Check sheet for the modelled part. Datum: model origin and axes. Units: mm. Face numbers are marked on the shaded views. A direction names the side the tool comes from. Give positions to 0.01 mm unless a question says otherwise; leave off trailing zeros. Order: outer loops, then holes, each group sorted by start corner. A loop starts at its lowest first (then second) coordinate and runs counter-clockwise, first axis right, second up.
from build123d import *

# Parameters (mm, degrees)
F0_R      = 2.25
F0_R_2    = 1
F1_DEPTH  = 4
F2_W      = 12
F2_H      = 12
F2_R      = 2.25
F3_DEPTH  = 6
F4_W      = 8
F4_H      = 8
F5_DEPTH  = 2
F6_R      = 4
F6_R_2    = 2.25
F7_DEPTH  = 5
F8_R      = 2.5
F8_R_2    = 1
F9_DEPTH  = 4
F11_DEPTH = 4.001


with BuildPart() as f1:
    # F0 (on Top) → F1 (new body)
    with BuildSketch(Plane.XY):
        Polygon((-30, 46), (-42, 46), (-42, -46), (-30, -46), (-30, -34), (13, -34), (13, -46), (25, -46), (25, -34), (40, -34), (40, 34), (25, 34), (25, 46), (13, 46), (13, 34), (-30, 34), align=None)
        with Locations((-36, -40)):
            Circle(F0_R, mode=Mode.SUBTRACT)
        with Locations((-30, -28)):
            Circle(F0_R_2, mode=Mode.SUBTRACT)
        with Locations((19, -40)):
            Circle(F0_R, mode=Mode.SUBTRACT)
        with Locations((28, -28)):
            Circle(F0_R_2, mode=Mode.SUBTRACT)
        with Locations((-30, 21)):
            Circle(F0_R_2, mode=Mode.SUBTRACT)
        with Locations((-36, 40)):
            Circle(F0_R, mode=Mode.SUBTRACT)
        with Locations((28, 21)):
            Circle(F0_R_2, mode=Mode.SUBTRACT)
        with Locations((19, 40)):
            Circle(F0_R, mode=Mode.SUBTRACT)
    extrude(amount=F1_DEPTH)

    # F2 (on face) → F3 (join)
    with BuildSketch(Plane.XY.offset(4)):
        with Locations((-36, -40)):
            Rectangle(F2_W, F2_H)
        with Locations((-36, -40)):
            Circle(F2_R, mode=Mode.SUBTRACT)
        with Locations((-36, 40)):
            Rectangle(F2_W, F2_H)
        with Locations((-36, 40)):
            Circle(F2_R, mode=Mode.SUBTRACT)
        with Locations((19, 40)):
            Rectangle(F2_W, F2_H)
        with Locations((19, 40)):
            Circle(F2_R, mode=Mode.SUBTRACT)
        with Locations((19, -40)):
            Rectangle(F2_W, F2_H)
        with Locations((19, -40)):
            Circle(F2_R, mode=Mode.SUBTRACT)
    extrude(amount=F3_DEPTH)

    # F4 (on face) → F5 (cut)
    with BuildSketch(Plane.XY.offset(10)):
        with Locations((-36, 40)):
            Rectangle(F4_W, F4_H)
        with Locations((19, 40)):
            Rectangle(F4_W, F4_H)
        with Locations((19, -40)):
            Rectangle(F4_W, F4_H)
        with Locations((-36, -40)):
            Rectangle(F4_W, F4_H)
    extrude(amount=-F5_DEPTH, mode=Mode.SUBTRACT)

    # F6 (on face) → F7 (cut)
    with BuildSketch(Plane(origin=(0, 0, 0), x_dir=(1, 0, 0), z_dir=(0, 0, -1))):
        with Locations((-36, 40)):
            Circle(F6_R)
        with Locations((-36, 40)):
            Circle(F6_R_2, mode=Mode.SUBTRACT)
        with Locations((19, 40)):
            Circle(F6_R)
        with Locations((19, 40)):
            Circle(F6_R_2, mode=Mode.SUBTRACT)
        with Locations((19, -40)):
            Circle(F6_R)
        with Locations((19, -40)):
            Circle(F6_R_2, mode=Mode.SUBTRACT)
        with Locations((-36, -40)):
            Circle(F6_R)
        with Locations((-36, -40)):
            Circle(F6_R_2, mode=Mode.SUBTRACT)
    extrude(amount=-F7_DEPTH, mode=Mode.SUBTRACT)

    # F8 (on face) → F9 (join)
    with BuildSketch(Plane.XY.offset(4)):
        with Locations((-30, 21)):
            Circle(F8_R)
        with Locations((-30, 21)):
            Circle(F8_R_2, mode=Mode.SUBTRACT)
        with Locations((-30, -28)):
            Circle(F8_R)
        with Locations((-30, -28)):
            Circle(F8_R_2, mode=Mode.SUBTRACT)
        with Locations((28, -28)):
            Circle(F8_R)
        with Locations((28, -28)):
            Circle(F8_R_2, mode=Mode.SUBTRACT)
        with Locations((28, 21)):
            Circle(F8_R)
        with Locations((28, 21)):
            Circle(F8_R_2, mode=Mode.SUBTRACT)
    extrude(amount=F9_DEPTH)

    # F10 (on face) → F11 (cut, through all)
    with BuildSketch(Plane.XY.offset(4)):
        with BuildLine():
            ThreePointArc((-36, 29.75), (-34.40901, 29.09099), (-33.75, 27.5))
            ThreePointArc((-33.75, 27.5), (-34.40901, 25.90901), (-36, 25.25))
            Line((-36, 25.25), (34, 25.25))
            ThreePointArc((34, 25.25), (31.75, 27.5), (34, 29.75))
            Line((34, 29.75), (-36, 29.75))
        make_face()
        with BuildLine():
            ThreePointArc((-36, 25.25), (-34.40901, 25.90901), (-33.75, 27.5))
            ThreePointArc((-33.75, 27.5), (-34.40901, 29.09099), (-36, 29.75))
            ThreePointArc((-36, 29.75), (-38.25, 27.5), (-36, 25.25))
        make_face()
        with BuildLine():
            ThreePointArc((-38.25, 16), (-36, 13.75), (-33.75, 16))
            ThreePointArc((-33.75, 16), (-36, 18.25), (-38.25, 16))
        make_face()
        with BuildLine():
            Line((-33.75, -23), (-33.75, 16))
            ThreePointArc((-33.75, 16), (-36, 13.75), (-38.25, 16))
            Line((-38.25, 16), (-38.25, -23))
            ThreePointArc((-38.25, -23), (-36, -20.75), (-33.75, -23))
        make_face()
        with BuildLine():
            ThreePointArc((-38.25, -23), (-36, -25.25), (-33.75, -23))
            ThreePointArc((-33.75, -23), (-36, -20.75), (-38.25, -23))
        make_face()
        with BuildLine():
            ThreePointArc((-23.752473, -19.972448), (-23.06584, -19.172576), (-22.818894, -18.147746))
            ThreePointArc((-22.818894, -18.147746), (-24.044064, -16.144693), (-26.385315, -16.323045))
            ThreePointArc((-26.385315, -16.323045), (-26.893596, -19.464167), (-23.752473, -19.972448))
        make_face()
        with BuildLine():
            ThreePointArc((-26.385315, -16.323045), (-24.044064, -16.144693), (-22.818894, -18.147746))
            ThreePointArc((-22.818894, -18.147746), (-23.06584, -19.172576), (-23.752473, -19.972448))
            Line((-23.752473, -19.972448), (23.579985, 14.175298))
            ThreePointArc((23.579985, 14.175298), (20.438863, 14.683579), (20.947143, 17.824702))
            Line((20.947143, 17.824702), (-26.385315, -16.323045))
        make_face()
        with BuildLine():
            ThreePointArc((24.513564, 16), (23.288394, 18.003054), (20.947143, 17.824702))
            ThreePointArc((20.947143, 17.824702), (20.438863, 14.683579), (23.579985, 14.175298))
            ThreePointArc((23.579985, 14.175298), (24.266618, 14.97517), (24.513564, 16))
        make_face()
        with BuildLine():
            ThreePointArc((36.25, 27.5), (35.59099, 29.09099), (34, 29.75))
            ThreePointArc((34, 29.75), (31.75, 27.5), (34, 25.25))
            ThreePointArc((34, 25.25), (35.59099, 25.90901), (36.25, 27.5))
        make_face()
        with BuildLine():
            Line((36.25, -23), (36.25, 16))
            ThreePointArc((36.25, 16), (34, 13.75), (31.75, 16))
            Line((31.75, 16), (31.75, -23))
            ThreePointArc((31.75, -23), (34, -20.75), (36.25, -23))
        make_face()
        with BuildLine():
            ThreePointArc((31.75, 16), (34, 13.75), (36.25, 16))
            ThreePointArc((36.25, 16), (34, 18.25), (31.75, 16))
        make_face()
        with BuildLine():
            ThreePointArc((31.75, -23), (34, -25.25), (36.25, -23))
            ThreePointArc((36.25, -23), (34, -20.75), (31.75, -23))
        make_face()
        with BuildLine():
            ThreePointArc((21.25, -28), (20.59099, -26.40901), (19, -25.75))
            ThreePointArc((19, -25.75), (16.75, -28), (19, -30.25))
            ThreePointArc((19, -30.25), (20.59099, -29.59099), (21.25, -28))
        make_face()
        with BuildLine():
            ThreePointArc((-21, -25.75), (-19.40901, -26.40901), (-18.75, -28))
            ThreePointArc((-18.75, -28), (-19.40901, -29.59099), (-21, -30.25))
            Line((-21, -30.25), (19, -30.25))
            ThreePointArc((19, -30.25), (16.75, -28), (19, -25.75))
            Line((19, -25.75), (-21, -25.75))
        make_face()
        with BuildLine():
            ThreePointArc((-21, -30.25), (-19.40901, -29.59099), (-18.75, -28))
            ThreePointArc((-18.75, -28), (-19.40901, -26.40901), (-21, -25.75))
            ThreePointArc((-21, -25.75), (-23.25, -28), (-21, -30.25))
        make_face()
    extrude(amount=-F11_DEPTH, mode=Mode.SUBTRACT)


solid = f1.part
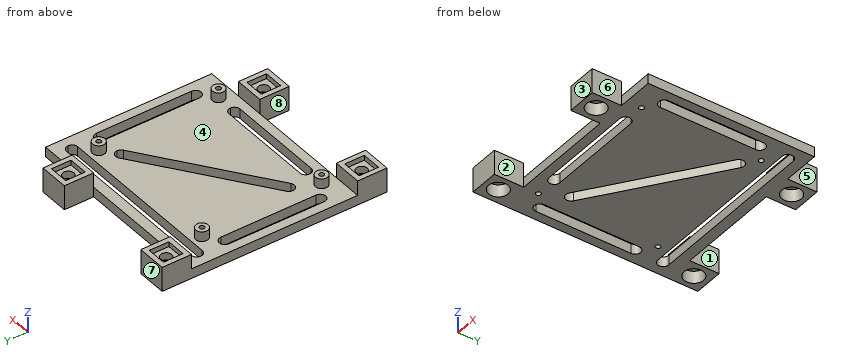
1) Material ranges on L1, parallel to Y at x = 19, z = 9.25; L2, parallel to Y at x = -36, z = 7.35; L3, parallel to X at y = 40, z = 5.6, recorded low to high.
Recorded:
L1: y = -46 to -44, -36 to -34, 34 to 36, 44 to 46
L2: y = -46 to -42.25, -37.75 to -34, 34 to 37.75, 42.25 to 46
L3: x = -42 to -38.25, -33.75 to -30, 13 to 16.75, 21.25 to 25
2) Draft check along X on the marked faces 6, 7 and 8. Enter one of: +X half, -X half, draft (parallel to the pull), parting line (faces both ways), or undercut.
Recorded:
face 6: +X half
face 7: draft
face 8: undercut
3) Section check B-B, the plane y = 21. Record the cut outline in (x, z).
Recorded:
outline: (-42, 0) - (-31, 0) - (-31, 8) - (-32.5, 8) - (-32.5, 4) - (-42, 4) - close; (-29, 0) - (27, 0) - (27, 8) - (25.5, 8) - (25.5, 4) - (-27.5, 4) - (-27.5, 8) - (-29, 8) - close; (29, 0) - (40, 0) - (40, 4) - (30.5, 4) - (30.5, 8) - (29, 8) - close
4) Section check A-A, the plane x = 28. Record the cut outline in (y, z), then the cut area to 3 significant figures.
Recorded:
outline: (-34, 0) - (-29, 0) - (-29, 8) - (-30.5, 8) - (-30.5, 4) - (-34, 4) - close; (-27, 0) - (20, 0) - (20, 8) - (18.5, 8) - (18.5, 4) - (-25.5, 4) - (-25.5, 8) - (-27, 8) - close; (22, 0) - (25.25, 0) - (25.25, 4) - (23.5, 4) - (23.5, 8) - (22, 8) - close; (29.75, 0) - (34, 0) - (34, 4) - (29.75, 4) - close
area: 262 mm2
5) Section check C-C, the plane y = 40. State how many separate pieces and enclosed holes the cut face has, then the cut area to 3 significant figures.
Recorded:
separate pieces: 4
enclosed holes: 0
area: 101 mm2
6) Depth check by flat-ended pin: pin 1 Ø5 at (x, y) = (-1.5, -8.5) entering from +Z; pin 2 Ø6 at (x, y) = (19, 40) entering from +Z; pin 3 Ø6 at (x, y) = (-36, 40) entering from -Z. Enter the tip coordinate at first touch or a pass-through.
Recorded:
pin 1: stops at z = 4
pin 2: stops at z = 8
pin 3: stops at z = 5
7) Section check D-D, the plane x = -12.5. Record the cut outline in (y, z), then the cut area to 3 significant figures.
Recorded:
outline: (-34, 0) - (-30.25, 0) - (-30.25, 4) - (-34, 4) - close; (-25.75, 0) - (-11.85, 0) - (-11.85, 4) - (-25.75, 4) - close; (-6.31, 0) - (25.25, 0) - (25.25, 4) - (-6.31, 4) - close; (29.75, 0) - (34, 0) - (34, 4) - (29.75, 4) - close
area: 214 mm2
8) Set-up check for the marked faces 1, 2, 3, 4 and 5: record each of +Z, -Z, +X, -X, +Y, -Y from which the full face is reachable in a straight line by a thin tool's end or side.
Recorded:
face 1: +Z, -Z, +Y
face 2: +Z, -Z, -Y
face 3: +Z, -Z, +X, -X, -Y
face 4: +Z
face 5: +Z, -Z, +X, +Y
